Autodesk Inventor part; units mm, degrees
ref_plane "YZ Plane" through (0, 0, 0) normal (1, 0, 0) x (0, 1, 0)
ref_plane "XZ Plane" through (0, 0, 0) normal (0, 1, 0) x (-1, 0, 0)
ref_plane "XY Plane" through (0, 0, 0) normal (0, 0, 1) x (1, 0, 0)
sketch "Sketch1" plane through (0, 0, 0) normal (0, 0, 1) x (1, 0, 0)
  line L0 (0, 0) -> (200, 0)
  line L1 (200, 0) -> (200, 10)
  line L2 (200, 10) -> (0, 10)
  line L3 (0, 10) -> (0, 0)
  dimension "d0" = 10
  dimension "d1" = 200
revolve "Revolution1" add sketch "Sketch1" angle 360 about axis through (0, 0, 0) along (1, 0, 0)
sketch "Sketch2" plane through (200, 0, 0) normal (1, 0, 0) x (0, 0, -1)
  line L0 (0, 17.3205) -> (15, 8.6603)
  line L1 (15, 8.6603) -> (15, -8.6603)
  line L2 (15, -8.6603) -> (0, -17.3205)
  line L3 (0, -17.3205) -> (-15, -8.6603)
  line L4 (-15, -8.6603) -> (-15, 8.6603)
  line L5 (-15, 8.6603) -> (0, 17.3205)
  point P0 (0, 0)
  point P1 (0, 0)
  dimension "d3" = 15
extrude "Extrusion1" add sketch "Sketch2" along normal blind 16
sketch "Sketch3" plane through (0, 0, 0) normal (0, 0, 1) x (1, 0, 0)
  line L0 (203.9505, 24.4808) -> (221.3427, 24.4808)
  line L1 (221.3427, 24.4808) -> (221.3427, 6.4675)
  line L2 (221.3427, 6.4675) -> (203.9505, 24.4808)
  line L3 (-22.4415, 0) -> (345.1219, 0) construction
  point P0 (0, 0)
revolve "Revolution2" cut sketch "Sketch3" angle 360 about axis through (-22.4415, 0, 0) along (1, 0, 0)
thread "Thread1"
properties part number "bolt M20x200"
Geometry check sheet. Reference: the model listing, model coordinates, mm. A direction names the side the tool comes from. Give positions to 0.01 mm unless a question says otherwise; leave off trailing zeros. Write each loop counter-clockwise with the first axis right and the second up, starting at its lowest first coordinate (ties: lowest second). Pieces come first, ordered by that corner, then holes. Notation, with made-up numbers: (-2, -3.75) -> (4, -3.75) arc R25 ccw to (4, 22.25) -> close; hole circle Ø6 at (49, 37). An arc over 180 degrees is marked (long way). Use one line per item in the form item = value.
Item 1: Sectioned sample at B-B on x = 71. Enter the section's corners in (y, z).
Results list:
outline = circle Ø20 at (0, 0)
Item 2: Sectioned sample at A-A on y = 0. Enter the section's corners in (x, z), plus the area to 3 significant figures.
Results list:
outline = (0, -10) -> (200, -10) -> (200, -15) -> (213.1, -15) -> (216, -12) -> (216, 12) -> (213.1, 15) -> (200, 15) -> (200, 10) -> (0, 10) -> close
area = 4,470 mm2
Item 3: Scan lines: line 1 (X direction, y = -10, z = 2.5); line 2 (Z direction, x = 108.5, y = -5); line 3 (X direction, y = -7.5, z = -12). Record each from-to range of solid material in increasing order.
Results list:
line_1 = 200 to 216
line_2 = -8.66 to 8.66
line_3 = 200 to 213.92
Item 4: Access from +Z, -Z, +X, -X, +Y, -Y to the whole of each face (thin tool, end or side, straight path). Record for faces 1 (the cylindrical face through (98.6, -2.17, 9.76)), 2 (the flat face through (206.46, -12.93, -7.605)).
Results list:
face_1 = -X
face_2 = -Z, +X, -X, -Y
Item 5: Depth check by flat-ended pin: pin 1 Ø3 at (x, z) = (116.5, -4.5) entering from +Y; pin 2 Ø2 at (y, z) = (12.5, 5) entering from -X; pin 3 Ø1.5 at (x, z) = (141, 6) entering from +Y. Enter the tip coordinate at first touch or a pass-through.
Results list:
pin_1 = 9.54
pin_2 = 200
pin_3 = 8.51
Item 6: Mould release check, pull along X, two halves, no side actions. Record for faces 3 (the flat face through (200, -7.5, 6.9)), 4 (the flat face through (206, 0, -15)), 5 (the flat face through (216, 0, 0)): released by +X, released by -X, zero draft, split by the parting line, or undercut.
Results list:
face_3 = released by -X
face_4 = zero draft
face_5 = released by +X
